Can you work these out from the model? Positions are in its coordinate system, mm. Face numbers are marked on the shaded views. A direction names the side the tool comes from. Give positions to 0.01 mm unless a question says otherwise; leave off trailing zeros. Write each loop counter-clockwise with the first axis right and the second up, starting at its lowest first coordinate (ties: lowest second). Pieces come first, ordered by that corner, then holes.
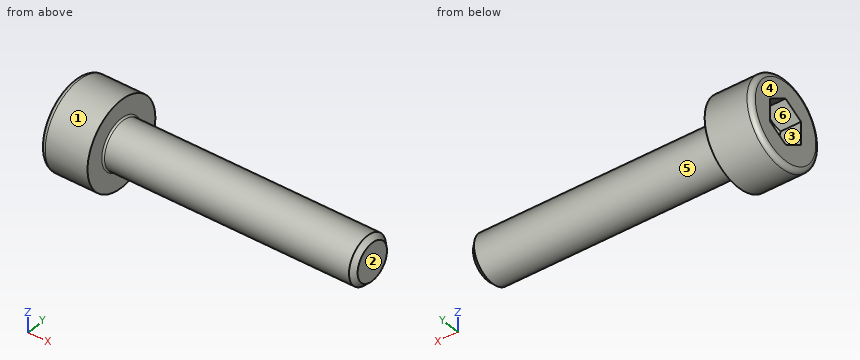
Autodesk Inventor part; units mm, degrees
ref_plane "Work Plane1" through (29, 0, 0) normal (0, -1, 0) x (1, 0, 0)
ref_plane "YZ Plane" through (0, 0, 0) normal (1, 0, 0) x (0, 1, 0)
ref_plane "XZ Plane" through (0, 0, 0) normal (0, 1, 0) x (-1, 0, 0)
sketch "Sketch1" plane through (0, 0, 0) normal (0, 0, 1) x (1, 0, 0)
  line L0 (-0.8667, 0) -> (16, 0)
  line L1 (16, 0) -> (16, 1.5)
  line L2 (16, 1.5) -> (12.25, 1.5)
  line L3 (12.25, 1.5) -> (11.9432, 1.5)
  line L4 (11.9432, 1.5) -> (0, 1.5)
  line L5 (0, 1.5) -> (0, 2.75)
  line L6 (0, 2.75) -> (-3, 2.75)
  line L7 (-3, 2.75) -> (-3, 1.4434)
  line L8 (-3, 1.4434) -> (-1.7, 1.4434)
  line L9 (-1.7, 1.4434) -> (-0.8667, 0)
  line L10 (-6.8, 0) -> (19.8, 0)
  line L11 (0, -0.55) -> (0, 3.3)
  line L12 (12.25, 1.5) -> (0, 1.5) construction
  dimension "d1" = 3.75
  dimension "d2" = 0.3068
  dimension "d3" = 3
  dimension "d4" = 1.3
  dimension "d5" = 60
  dimension "d6" = 3
  dimension "d7" = 3
  dimension "d8" = 2.8868
  dimension "d9" = 5.5
  dimension "d26" = 16
revolve "Body" add sketch "Sketch1" angle 360 about axis through (-0.8667, 0, 0) along (1, 0, 0)
sketch "Sketch2" plane through (-3, 0, 0) normal (-1, 0, 0) x (0, 0, 1)
  circle A0 centre (0, 0) radius 1.4434
  line L0 (0, -3.85) -> (0, 3.85)
  line L1 (-3.85, 0) -> (3.85, 0)
  line L2 (1.4434, 0) -> (0.7217, -1.25)
  line L3 (0.7217, -1.25) -> (-0.7217, -1.25)
  line L4 (-0.7217, -1.25) -> (-1.4434, 0)
  line L5 (-1.4434, 0) -> (-0.7217, 1.25)
  line L6 (-0.7217, 1.25) -> (0.7217, 1.25)
  line L7 (0.7217, 1.25) -> (1.4434, 0)
  point P0 (0, 0)
extrude "Slot" add sketch "Sketch2" against normal up to next contours L7 A0 | A0 L2 | L6 L0 A0 | A0 L0 L3 | L0 L6 A0 | A0 L3 L0 | L4 A0 | A0 L5
fillet "Fillet1" radius 0.3 1 edges at (-3, -2.75, 0)
thread "Thread"
chamfer "Chamfer1" distance 0.3067 distance2 0.3067 1 edges at (16, -1.5, 0) measured on face at (16, -0.4645, -0.4115)
ref_plane "Work Plane1" through (29, 0, 0) normal (0, -1, 0) x (1, 0, 0)
fillet "Fillet2" radius 0.1 1 edges at (0, -1.5, 0)
equation "\"d1\" = GEL"
equation "\"d3\" = KOH"
equation "\"d4\" = INTI"
equation "\"d6\" = GD"
equation "\"d7\" = BDM"
equation "\"d8\" = 1.1547 * SW"
equation "\"d9\" = KOD"
equation "\"d30\" = R"
equation "\"d17\" = RR"
equation "\"d15\" = -0.5 * SPD + 0.5 * GD"
equation "\"d16\" = GUL"
equation "\"GD\" = 3"
equation "\"NLG\" = 5"
equation "\"GEL\" = 3.75"
equation "\"KOD\" = 5.5"
equation "\"KOH\" = 3"
equation "\"INTI\" = 1.3"
equation "\"GAL\" = 0.61345 * PTC"
equation "\"GUL\" = 0.61345 * PTC"
equation "\"BDM\" = NND"
equation "\"SW\" = 2.5"
equation "\"RR\" = 0.3"
equation "\"SPD\" = NND - 1.2269 * PTC"
equation "\"R\" = 0.1"
equation "\"TOA\" = 30deg"
equation "\"GD1\" = THREADDIA - 1.2269 * PTC"
equation "\"THREADDIA\" = 3"
equation "\"FAWI\" = 45deg"
equation "\"PTC\" = 0.5"
equation "\"NND\" = 3"
equation "\"E0\" = 1.155 * SW"
properties part number "Allen Key 3x16mm" material "Stainless Steel, 440C"
(1) Imagine slicing it at B-B, the plane x = 9. Write out the boundary of the cut face in (y, z).
Returned:
outline: circle Ø3 at (0, 0)
(2) Imagine slicing it at A-A, the plane x = -2. Write out the boundary of the cut face in (y, z).
Returned:
outline: circle Ø5.5 at (0, 0); hole (-1.25, -0.72) - (0, -1.44) - (1.25, -0.72) - (1.25, 0.72) - (0, 1.44) - (-1.25, 0.72) - close
(3) If I drill on L1, parallel to X at y = 1.95, z = -0.65; L2, parallel to Z at x = 12, y = -0.05; L3, parallel to Z at x = -0.5, y = 0.15, over which ranges is the centre line in solid material (lowest first)?
Returned:
L1: x = -3 to 0
L2: z = -1.5 to 1.5
L3: z = -2.75 to 2.75
(4) If we mould it in two halves opening along Y, with no side actions, what happens to the marked faces 1, 2 and 3? For each: +Y half, -Y half, draft (parallel to the pull), parting line (faces both ways), or undercut.
Returned:
face 1: parting line
face 2: draft
face 3: undercut
(5) For the marked faces 4, 5 and 6, which set-ups out of +Z, -Z, +X, -X, +Y, -Y let a thin tool reach every point of the face, with its end or its side?
Returned:
face 4: +Z, -Z, -X, +Y, -Y
face 5: +X
face 6: -X
(6) Will these pins go through, and if not, where does the flat tip stop? P1, Ø1.5, axis at x = 6.5, z = -2, coming from the +Y side; P2, Ø1, axis at x = 4, y = 0, coming from the -Z side; P3, Ø2, axis at x = 5.5, z = 1, coming from the -Y side.
Returned:
P1: stops at y = 0.83
P2: stops at z = -1.5
P3: stops at y = -1.5
